```python
from build123d import *

# Parameters (mm, degrees)
ESQUISSE1_R      = 28.5
EXTRUSION1_DEPTH = 5
ESQUISSE2_R      = 7.5
EXTRUSION2_DEPTH = 5
EXTRUSION3_REACH = 12
ESQUISSE3_R      = 2
ESQUISSE12_W     = 1.25
ESQUISSE12_H     = 28.5


with BuildPart() as part:
    # Esquisse1 → Extrusion1 (new body)
    with BuildSketch(Plane.XY):
        Circle(ESQUISSE1_R)
    extrude(amount=-EXTRUSION1_DEPTH)

    # Esquisse2 → Extrusion2 (add)
    with BuildSketch(Plane.XY):
        Circle(ESQUISSE2_R)
    extrude(amount=EXTRUSION2_DEPTH)

    # Esquisse3 → Extrusion3 (cut, up to next)
    with BuildSketch(Plane.XY.offset(5), mode=Mode.PRIVATE) as extrusion3_sk1:
        Circle(ESQUISSE3_R)
    extrusion3_tool1 = extrude(extrusion3_sk1.sketch, amount=-EXTRUSION3_REACH, mode=Mode.PRIVATE) & part.part
    add(extrusion3_tool1.solids().sort_by_distance((0, 0, 5))[0], mode=Mode.SUBTRACT)

    # Esquisse6 → Enlèvement de matière-Révolution3 (revolve, cut)
    with BuildSketch(Plane(origin=(0, 0, 0), x_dir=(1, 0, 0), z_dir=(0, 1, 0))):
        with BuildLine():
            Line((-29, 4.5), (-31.449617094, 4.5))
            Line((-31.449617094, 4.5), (-31.449617094, 0.5))
            Line((-31.449617094, 0.5), (-29, 0.5))
            ThreePointArc((-29, 0.5), (-27, 2.5), (-29, 4.5))
        make_face()
    revolve(axis=Axis((0, 0, 5), (0, 0, -1)), mode=Mode.SUBTRACT)

    # Esquisse12 → Trou taraudé M3x0.55 (revolve, cut)
    with BuildSketch(Plane(origin=(0, 0, 2.5), x_dir=(0, 0, 1), z_dir=(1, 0, 0))):
        with Locations((0.625, 14.25)):
            Rectangle(ESQUISSE12_W, ESQUISSE12_H)
    revolve(axis=Axis((0, 6.35, 2.5), (0, -1, 0)), mode=Mode.SUBTRACT)


solid = part.part
```
Here's how the part is built. I have some questions about the finished solid (model axes, mm). A direction names the side the tool comes from. Coordinates: 2 decimals unless noted, no trailing zeros. Write each loop counter-clockwise with the first axis right and the second up, starting at its lowest first coordinate (ties: lowest second). Pieces come first, ordered by that corner, then holes. Notation, with made-up numbers: M -4.5,87.25 L 49.5,87.25 A23 ccw 49.5,118.25 Z; hole C 57.5,19.25 d8. An arc over 180 degrees is marked long. Answer as CSV lines item,"result". Start each with the question number.
Q1. If we mould it in two halves opening along X, with no side actions, what happens to faces 4 (the cylindrical face through (15.32, 24.03, -4.71)), 5 (the cylindrical face through (0, 2, 0)), 6 (the flat face through (2, -2, 5))? For each: pulls with the +X half, pulls with the -X half, needs draft (parallel to the pull), parting line crosses it, or undercut.
Q2. For faces 1 (the flat face through (6, -6, 0)), 2 (the cylindrical face through (15.32, 24.03, -0.28)), 3 (the cylindrical face through (-0.05, -4.57, 1.25)), which set-ups out of +Z, -Z, +X, -X, +Y, -Y let a thin tool reach every point of the face, with its end or its side?
Q3. Will these pins go through, and if not, where does the flat tip stop? pin 1 Ø2 at (y, z) = (-7, 0) entering from +X; pin 2 Ø1.5 at (x, y) = (15, -4) entering from +Z; pin 3 Ø1.5 at (x, z) = (0, 2.5) entering from +Y.
Q4. Suppose I cut it at D-D, the plane z = 2.5. List the corners of the cut face in (x, y) for me.
Q5. I need wall thicknesses on probe 1 along Z at (x, y) = (0, -3.25); probe 2 along X at (y, z) = (-5.8, 2.5) (3 decimals); probe 3 along Y at (x, z) = (0.5, 0.75). Which ranges of each line are inside material? Lowest first, please. Write a range as [from, to].
Q6. Suppose I cut it at A-A, the plane x = 0. List the corners of the cut face in (y, z) for me.
Q7. Suppose I cut it at C-C, the plane z = -3.75. List the corners of the cut face in (x, y) for me, then the cut area to 3 significant figures.
Q8. Suppose I cut it at B-B, the plane y = 0. List the corners of the cut face in (x, z) for me.
Entries:
1,face 4,"parting line crosses it"
1,face 5,"undercut"
1,face 6,"needs draft"
2,face 1,"+Z"
2,face 2,"+Z, -Z"
2,face 3,"-Y"
3,pin 1,"stops at x = 27.86"
3,pin 2,"stops at z = 0"
3,pin 3,"stops at y = 7.5"
4,outline,"M -1.25,-7.4 L -1.25,-1.56 A2 cw long 1.25,-1.56 L 1.25,-7.4 A7.5 ccw long Z"
5,probe 1,"z = [-5, 1.25], [3.75, 5]"
5,probe 2,"x = [-4.755, -1.25], [1.25, 4.755]"
5,probe 3,"y = [-7.48, -1.94], [1.94, 7.48]"
6,outline,"M -28.5,-5 L -2,-5 L -2,1.25 L -7.5,1.25 L -7.5,0 L -28.5,0 L -28.5,-0.56 A2 cw -28.5,-4.44 Z; M -7.5,3.75 L -2,3.75 L -2,5 L -7.5,5 Z; M 2,-5 L 28.5,-5 L 28.5,-4.44 A2 cw 28.5,-0.56 L 28.5,0 L 7.5,0 L 7.5,5 L 2,5 Z"
7,outline,"C 0,0 d54.88; hole C 0,0 d4"
7,area,"2,350 mm²"
8,outline,"M -28.5,-5 L -2,-5 L -2,5 L -7.5,5 L -7.5,0 L -28.5,0 L -28.5,-0.56 A2 cw -28.5,-4.44 Z; M 2,-5 L 28.5,-5 L 28.5,-4.44 A2 cw 28.5,-0.56 L 28.5,0 L 7.5,0 L 7.5,5 L 2,5 Z"
